from build123d import *

# Parameters (mm, degrees)
SKETCH1_W           = 12
SKETCH1_H           = 27
SKETCH1_R           = 1.5
SKETCH1_R_2         = 3
BOSS_EXTRUDE1_DEPTH = 12
BOSS_EXTRUDE2_START = 12
SKETCH1_3_W         = 32
SKETCH1_3_H         = 27
SKETCH1_3_R         = 1.5
SKETCH1_3_R_2       = 3
BOSS_EXTRUDE2_DEPTH = 3
SKETCH2_3_R         = 1.5
CUT_EXTRUDE2_DEPTH  = 29.41214529
SKETCH3_W           = 15
SKETCH3_H           = 1.5
SKETCH3_R           = 1.5
BOSS_EXTRUDE3_DEPTH = 12
SKETCH3_4_R         = 1.5
CUT_EXTRUDE3_DEPTH  = 9
SKETCH3_5_R         = 1.5
CUT_EXTRUDE4_DEPTH  = 41.607881008
CUT_EXTRUDE9_START  = 3
SKETCH1_4_R         = 3
SKETCH1_4_R_2       = 1.5
CUT_EXTRUDE9_DEPTH  = 9
SKETCH4_W           = 3
SKETCH4_H           = 26.5
SKETCH4_W_2         = 5
SKETCH4_H_2         = 26
BOSS_EXTRUDE4_DEPTH = 5
SKETCH4_3_W         = 3
SKETCH4_3_H         = 26.5
BOSS_EXTRUDE5_DEPTH = 25
SKETCH5_W           = 3
SKETCH5_H           = 27
BOSS_EXTRUDE6_DEPTH = 10
CUT_EXTRUDE10_REACH = 56.658
SKETCH6_R           = 1.5
SKETCH7_R           = 2.5
SKETCH7_R_2         = 1.5
BOSS_EXTRUDE7_DEPTH = 0.5
BOSS_EXTRUDE8_START = 9.3
SKETCH7_2_R         = 2.5
SKETCH7_2_R_2       = 1.5
BOSS_EXTRUDE8_DEPTH = 0.5
SKETCH2_R           = 3
SKETCH2_R_2         = 1.5
CUT_EXTRUDE1_DEPTH  = 41.193158622
SKETCH8_W           = 9.3
SKETCH8_H           = 20
BOSS_EXTRUDE9_DEPTH = 1.5


with BuildPart() as part:
    # Sketch1 → Boss-Extrude1 (new body)
    with BuildSketch(Plane.XY):
        with Locations((-10, 0)):
            Rectangle(SKETCH1_W, SKETCH1_H)
        with Locations(Location((-10, 10, 0), (0, 0, 90))):
            Circle(SKETCH1_R, mode=Mode.SUBTRACT)
        with Locations(Location((-10, -10, 0), (0, 0, 90))):
            Circle(SKETCH1_R, mode=Mode.SUBTRACT)
        with Locations((10, 0)):
            Rectangle(SKETCH1_W, SKETCH1_H)
        with Locations((10, 10)):
            Circle(SKETCH1_R_2, mode=Mode.SUBTRACT)
        with Locations(Location((10, -10, 0), (0, 0, 90))):
            Circle(SKETCH1_R, mode=Mode.SUBTRACT)
        with Locations((10, 10)):
            Circle(SKETCH1_R_2)
        with Locations(Location((10, 10, 0), (0, 0, 90))):
            Circle(SKETCH1_R, mode=Mode.SUBTRACT)
        with Locations((-10, 10)):
            Circle(SKETCH1_R_2)
        with Locations(Location((-10, 10, 0), (0, 0, 90))):
            Circle(SKETCH1_R, mode=Mode.SUBTRACT)
    extrude(amount=BOSS_EXTRUDE1_DEPTH)

    # Sketch1_3 → Boss-Extrude2 (add)
    with BuildSketch(Plane.XY.offset(BOSS_EXTRUDE2_START)):
        Rectangle(SKETCH1_3_W, SKETCH1_3_H)
        with Locations(Location((-10, -10, 0), (0, 0, 90))):
            Circle(SKETCH1_3_R, mode=Mode.SUBTRACT)
        with Locations(Location((-10, 10, 0), (0, 0, 90))):
            Circle(SKETCH1_3_R_2, mode=Mode.SUBTRACT)
        with Locations(Location((10, 10, 0), (0, 0, 90))):
            Circle(SKETCH1_3_R_2, mode=Mode.SUBTRACT)
        with Locations(Location((10, -10, 0), (0, 0, 90))):
            Circle(SKETCH1_3_R, mode=Mode.SUBTRACT)
    extrude(amount=BOSS_EXTRUDE2_DEPTH)

    # Sketch2_3 → Cut-Extrude2 (cut, through all)
    with BuildSketch(Plane.ZY.offset(4)):
        with Locations((6, -15)):
            Circle(SKETCH2_3_R)
        with Locations(Location((6, 10, 0), (0, 0, 270))):
            Circle(SKETCH2_3_R)
    extrude(amount=-CUT_EXTRUDE2_DEPTH, mode=Mode.SUBTRACT)

    # Sketch3 → Boss-Extrude3 (add)
    with BuildSketch(Plane(origin=(16, 0, 0), x_dir=(0, 0, -1), z_dir=(1, 0, 0))):
        Polygon((-9, -13.5), (-15, -13.5), (-15, -20), (0, -20), (0, -13.5), (-3, -13.5), (-3, -16.732050808), (-6, -18.464101615), (-9, -16.732050808), align=None)
        with Locations((-7.5, 14.25)):
            Rectangle(SKETCH3_W, SKETCH3_H)
        Polygon((-6, -13.5), (-9, -13.5), (-9, -16.732050808), (-6, -18.464101615), (-3, -16.732050808), (-3, -13.5), align=None)
        with BuildLine():
            ThreePointArc((-4.5, -15), (-7.060660172, -16.060660172), (-6, -13.5))
            ThreePointArc((-6, -13.5), (-4.939339828, -13.939339828), (-4.5, -15))
        make_face(mode=Mode.SUBTRACT)
        with Locations((-6, -15)):
            Circle(SKETCH3_R)
    extrude(amount=-BOSS_EXTRUDE3_DEPTH)

    # Sketch3_4 → Cut-Extrude3 (cut)
    with BuildSketch(Plane(origin=(16, 0, 0), x_dir=(0, 0, -1), z_dir=(1, 0, 0))):
        Polygon((-6, 13.464101615), (-9, 11.732050808), (-9, 8.267949192), (-6, 6.535898385), (-3, 8.267949192), (-3, 11.732050808), align=None)
        Polygon((-6, -11.535898385), (-9, -13.267949192), (-9, -16.732050808), (-6, -18.464101615), (-3, -16.732050808), (-3, -13.267949192), align=None)
        with Locations(Location((-6, -15, 0), (0, 0, 90))):
            Circle(SKETCH3_4_R, mode=Mode.SUBTRACT)
    extrude(amount=-CUT_EXTRUDE3_DEPTH, mode=Mode.SUBTRACT)

    # Sketch3_5 → Cut-Extrude4 (cut, through all)
    with BuildSketch(Plane(origin=(16, 0, 0), x_dir=(0, 0, -1), z_dir=(1, 0, 0))):
        with Locations(Location((-6, -15, 0), (0, 0, 90))):
            Circle(SKETCH3_5_R)
        with Locations(Location((-6, 10, 0), (0, 0, 90))):
            Circle(SKETCH3_5_R)
    extrude(amount=-CUT_EXTRUDE4_DEPTH, mode=Mode.SUBTRACT)

    # Sketch1_4 → Cut-Extrude9 (cut)
    with BuildSketch(Plane.XY.offset(CUT_EXTRUDE9_START)):
        with Locations(Location((-10, 10, 0), (0, 0, 180))):
            Circle(SKETCH1_4_R)
        with Locations(Location((-10, 10, 0), (0, 0, 180))):
            Circle(SKETCH1_4_R_2, mode=Mode.SUBTRACT)
        with Locations(Location((10, 10, 0), (0, 0, 180))):
            Circle(SKETCH1_4_R)
        with Locations(Location((10, 10, 0), (0, 0, 180))):
            Circle(SKETCH1_4_R_2, mode=Mode.SUBTRACT)
    extrude(amount=CUT_EXTRUDE9_DEPTH, mode=Mode.SUBTRACT)

    # Sketch4 → Boss-Extrude4 (add)
    with BuildSketch(Plane.XY):
        with Locations((-26.8, 0.25)):
            Rectangle(SKETCH4_W, SKETCH4_H)
        Polygon((-25.3, -13), (-21, -13), (-21, 13), (-16, 13), (-16, 13.5), (-25.3, 13.5), align=None)
        with Locations((-18.5, 0)):
            Rectangle(SKETCH4_W_2, SKETCH4_H_2)
    extrude(amount=BOSS_EXTRUDE4_DEPTH)

    # Sketch4_3 → Boss-Extrude5 (add)
    with BuildSketch(Plane.XY):
        with Locations((-26.8, 0.25)):
            Rectangle(SKETCH4_3_W, SKETCH4_3_H)
    extrude(amount=BOSS_EXTRUDE5_DEPTH)

    # Sketch5 → Boss-Extrude6 (add)
    with BuildSketch(Plane.XY.offset(15)):
        with Locations((-14.5, 0)):
            Rectangle(SKETCH5_W, SKETCH5_H)
    extrude(amount=BOSS_EXTRUDE6_DEPTH)

    # Cut-Extrude10: up to this face of the body (flat: up to its plane)
    cut_extrude10_end = Plane(part.part.faces().sort_by_distance((-13, 0, 20))[0])
    # Sketch6 → Cut-Extrude10 (cut, up to the picked face)
    with BuildSketch(Plane.ZY.offset(28.3), mode=Mode.PRIVATE) as cut_extrude10_sk1:
        with Locations((16.04, 0.25)):
            Circle(SKETCH6_R)
    cut_extrude10_tool1 = split(extrude(cut_extrude10_sk1.sketch, amount=-CUT_EXTRUDE10_REACH, mode=Mode.PRIVATE), bisect_by=cut_extrude10_end, keep=Keep.BOTH, mode=Mode.PRIVATE)
    add(cut_extrude10_tool1.solids().sort_by(Axis((-28.3, 0.25, 16.04), (1, 0, 0)))[0], mode=Mode.SUBTRACT)

    # Sketch7 → Boss-Extrude7 (add)
    with BuildSketch(Plane(origin=(-25.3, 0, 0), x_dir=(0, 0, -1), z_dir=(1, 0, 0))):
        with Locations(Location((-16.04, 0.25, 0), (0, 0, 180))):
            Circle(SKETCH7_R)
        with Locations(Location((-16.04, 0.25, 0), (0, 0, 180))):
            Circle(SKETCH7_R_2, mode=Mode.SUBTRACT)
    extrude(amount=BOSS_EXTRUDE7_DEPTH)

    # Sketch7_2 → Boss-Extrude8 (add)
    with BuildSketch(Plane(origin=(-25.3, 0, 0), x_dir=(0, 0, -1), z_dir=(1, 0, 0)).offset(BOSS_EXTRUDE8_START)):
        with Locations(Location((-16.04, 0.25, 0), (0, 0, 180))):
            Circle(SKETCH7_2_R)
        with Locations(Location((-16.04, 0.25, 0), (0, 0, 180))):
            Circle(SKETCH7_2_R_2, mode=Mode.SUBTRACT)
    extrude(amount=-BOSS_EXTRUDE8_DEPTH)

    # Sketch2 → Cut-Extrude1 (cut, through all)
    with BuildSketch(Plane.ZY.offset(4)):
        with Locations((6, -15)):
            Circle(SKETCH2_R)
        with Locations(Location((6, -15, 0), (0, 0, 90))):
            Circle(SKETCH2_R_2, mode=Mode.SUBTRACT)
        with Locations(Location((6, 10, 0), (0, 0, 270))):
            Circle(SKETCH2_R)
        with Locations(Location((6, 10, 0), (0, 0, 90))):
            Circle(SKETCH2_R_2, mode=Mode.SUBTRACT)
        with Locations(Location((6, -15, 0), (0, 0, 90))):
            Circle(SKETCH2_R_2)
    extrude(amount=CUT_EXTRUDE1_DEPTH, mode=Mode.SUBTRACT)


with BuildPart() as cut_extrude1_kept_piece:
    # of the separate pieces the step leaves, the one the design keeps (cut_extrude1_pieces_kept)
    add(part.part.solids().sort_by_distance((-16, -13.5, 25))[0])

    # Sketch8 → Boss-Extrude9 (add)
    with BuildSketch(Plane(origin=(0, 13.5, 0), x_dir=(1, 0, 0), z_dir=(0, 1, 0))):
        Polygon((-28.3, -25), (-25.3, -25), (-25.3, -5), (-16, -5), (-16, -25), (-13, -25), (-13, -15), (4, -15), (4, -12), (-4, -12), (-4, 0), (-28.3, 0), align=None)
        with Locations((-20.65, -15)):
            Rectangle(SKETCH8_W, SKETCH8_H)
    extrude(amount=BOSS_EXTRUDE9_DEPTH)


solid = cut_extrude1_kept_piece.part
Check sheet for the modelled part. Datum: model origin and axes. Units: mm. A direction names the side the tool comes from. Round coordinates to 2 decimals unless told otherwise and drop trailing zeros. Order: outer loops, then holes, each group sorted by start corner. A loop starts at its lowest first (then second) coordinate and runs counter-clockwise, first axis right, second up.
Q1. Cross-section at B-B, the plane y = 0.25. Give the number of separate pieces and of enclosed holes in the cut face, plus the area to 4 significant figures.
Filled sheet:
separate pieces: 3
enclosed holes: 0
area: 519.5 mm2
Q2. Set-up check for faces 1 (the face through (-14.73, -0.2, 17.47)), 2 (the face through (11.6, -17.6, 4.5)), 3 (the face through (-10, 7, 4)), 4 (the face through (-16.247, 0.14, 13.542)): record each of +Z, -Z, +X, -X, +Y, -Y from which the full face is reachable in a straight line by a thin tool's end or side.
Filled sheet:
face 1: -X
face 2: +X
face 3: +Z
face 4: none
Q3. Cross-section at A-A, the plane x = 9.5. Enter the section's corners in (y, z), plus the area to 3 significant figures.
Filled sheet:
outline: (-20, 0) - (-11.41, 0) - (-11.41, 15) - (-20, 15) - close; (-8.59, 0) - (8.59, 0) - (8.59, 3) - (7.04, 3) - (7.04, 5.12) - (6.54, 6) - (7.04, 6.88) - (7.04, 15) - (-8.59, 15) - close; (11.41, 0) - (15, 0) - (15, 15) - (12.96, 15) - (12.96, 6.88) - (13.46, 6) - (12.96, 5.12) - (12.96, 3) - (11.41, 3) - close; hole (-18.46, 6) - (-16.73, 3) - (-13.27, 3) - (-11.54, 6) - (-13.27, 9) - (-16.73, 9) - close
area: 371 mm2
Q4. Depth check by flat-ended pin: P1, Ø8, axis at x = -11, z = 8.5, coming from the -Y side; P2, Ø3, axis at x = -20.5, z = 13.5, coming from the -Y side; P3, Ø2, axis at y = 8, z = 21.5, coming from the +X side. Enter the tip coordinate at first touch or a pass-through.
Filled sheet:
P1: stops at y = -13.5
P2: stops at y = 13.5
P3: stops at x = -13
Q5. Cross-section at D-D, the plane x = -5. Enter the section's corners in (y, z), plus the area to 3 significant figures.
Filled sheet:
outline: (-13.5, 0) - (15, 0) - (15, 15) - (-13.5, 15) - (-13.5, 8.6) arc R3 cw to (-13.5, 3.4) - close; hole circle Ø6 at (10, 6)
area: 394 mm2
Q6. Draft check along Y on faces 5 (the face through (-4, 1, 6)), 6 (the face through (-22, -13, 2)), 7 (the face through (12, 10, 3)). Enter one of: pulls with the +Y half, pulls with the -Y half, needs draft (parallel to the pull), parting line crosses it, or undercut.
Filled sheet:
face 5: needs draft
face 6: pulls with the -Y half
face 7: undercut
Q7. Scan lines: L1, parallel to X at y = -4, z = 7; L2, parallel to X at y = 10, z = 9.25; L3, parallel to X at y = 10, z = 1.85. Record each from-to range of solid material in increasing order.
Filled sheet:
L1: x = -28.3 to -25.3, -16 to -4, 4 to 16
L2: x = -28.3 to -25.3, -16 to -13, -7 to -4, 4 to 7, 13 to 16
L3: x = -28.3 to -11.5, -8.5 to -4, 4 to 8.5, 11.5 to 16
Q8. Cross-section at C-C, the plane x = -21.5. Enter the section's corners in (y, z).
Filled sheet:
outline: (-13, 0) - (15, 0) - (15, 25) - (13.5, 25) - (13.5, 5) - (12.83, 5) arc R3 cw to (7.17, 5) - (-12.17, 5) arc R3 cw to (-13, 3.76) - close
